The listing builds one solid part. Answer for the finished solid, in the listing's coordinates (mm). A direction names the side the tool comes from. Round coordinates to 2 decimals unless told otherwise and drop trailing zeros. Loops run counter-clockwise (first coordinate to the right, second up) from the corner with the lowest first, then second, coordinate; pieces in that order, holes last. Notation, with made-up numbers: (-35, 32.25) - (-14, 32.25) arc R29 ccw to (-14, 61.25) - close; hole circle Ø5 at (65, 47.25). An arc over 180 degrees is marked (long way). One line per item, written item: value.
```python
from build123d import *

# Parameters (mm, degrees)
F0_R     = 3
F0_R_2   = 1.5
F1_DEPTH = 25


with BuildPart() as f1:
    # F0 (on Front) → F1 (new body)
    with BuildSketch(Plane.XZ):
        with BuildLine():
            Line((14.5, 22.5), (-16.5, 22.5))
            ThreePointArc((-16.5, 22.5), (-17.9142135624, 21.9142135624), (-18.5, 20.5))
            Line((-18.5, 20.5), (-18.5, 17.6726558901))
            Line((-18.5, 17.6726558901), (-18.5, -20.5))
            ThreePointArc((-18.5, -20.5), (-17.9142135624, -21.9142135624), (-16.5, -22.5))
            Line((-16.5, -22.5), (-2.7271780287, -22.5))
            ThreePointArc((-2.7271780287, -22.5), (-3, -21.25), (-2.7271780287, -20))
            Line((-2.7271780287, -20), (-14, -20))
            ThreePointArc((-14, -20), (-14.7071067812, -19.7071067812), (-15, -19))
            Line((-15, -19), (-15, -15.5))
            Line((-15, -15.5), (-15, 2.5))
            ThreePointArc((-15, 2.5), (-14.4142135624, 3.9142135624), (-13, 4.5))
            Line((-13, 4.5), (-12, 4.5))
            ThreePointArc((-12, 4.5), (-10.5857864376, 5.0857864376), (-10, 6.5))
            Line((-10, 6.5), (-10, 8.1054256072))
            ThreePointArc((-10, 8.1054256072), (-9.6405519552, 9.2493614806), (-8.6914107177, 9.9821118409))
            Line((-8.6914107177, 9.9821118409), (6.3085892823, 15.5084276303))
            ThreePointArc((6.3085892823, 15.5084276303), (8.1439358734, 15.2722933519), (9, 13.6317413967))
            Line((9, 13.6317413967), (9, 2.5))
            ThreePointArc((9, 2.5), (9.2928932188, 1.7928932188), (10, 1.5))
            Line((10, 1.5), (13, 1.5))
            ThreePointArc((13, 1.5), (14.4142135624, 0.9142135624), (15, -0.5))
            Line((15, -0.5), (15, -15.5))
            ThreePointArc((15, -15.5), (14.9989931779, -15.5634529316), (14.9959737255, -15.6268419774))
            Line((14.9959737255, -15.6268419774), (14.8878943659, -19.0317264658))
            ThreePointArc((14.8878943659, -19.0317264658), (14.5841971496, -19.7182361958), (13.8883977769, -20))
            Line((13.8883977769, -20), (2.7271780287, -20))
            ThreePointArc((2.7271780287, -20), (2.9310010309, -20.6102868166), (3, -21.25))
            ThreePointArc((3, -21.25), (2.9310010309, -21.8897131834), (2.7271780287, -22.5))
            Line((2.7271780287, -22.5), (16.5, -22.5))
            ThreePointArc((16.5, -22.5), (17.9142135624, -21.9142135624), (18.5, -20.5))
            Line((18.5, -20.5), (18.5, 3.5))
            ThreePointArc((18.5, 3.5), (18.2071067812, 4.2071067812), (17.5, 4.5))
            ThreePointArc((17.5, 4.5), (16.7928932188, 4.7928932188), (16.5, 5.5))
            Line((16.5, 5.5), (16.5, 17.6726558901))
            Line((16.5, 17.6726558901), (16.5, 20.5))
            ThreePointArc((16.5, 20.5), (15.9142135624, 21.9142135624), (14.5, 22.5))
        make_face()
        with BuildLine():
            ThreePointArc((-12.5, 17.6726558901), (-15.5, 14.6726558901), (-18.5, 17.6726558901))
            ThreePointArc((-18.5, 17.6726558901), (-15.5, 20.6726558901), (-12.5, 17.6726558901))
        make_face(mode=Mode.SUBTRACT)
        with Locations((13.5, 17.6726558901)):
            Circle(F0_R, mode=Mode.SUBTRACT)
        with BuildLine():
            ThreePointArc((-2.7271780287, -20), (-3, -21.25), (-2.7271780287, -22.5))
            Line((-2.7271780287, -22.5), (-0.8291561976, -22.5))
            ThreePointArc((-0.8291561976, -22.5), (-1.5, -21.25), (-0.8291561976, -20))
            Line((-0.8291561976, -20), (-2.7271780287, -20))
        make_face()
        with BuildLine():
            Line((-0.8291561976, -22.5), (-2.7271780287, -22.5))
            ThreePointArc((-2.7271780287, -22.5), (0, -24.25), (2.7271780287, -22.5))
            Line((2.7271780287, -22.5), (0.8291561976, -22.5))
            ThreePointArc((0.8291561976, -22.5), (0, -22.75), (-0.8291561976, -22.5))
        make_face()
        with BuildLine():
            Line((0.8291561976, -22.5), (2.7271780287, -22.5))
            ThreePointArc((2.7271780287, -22.5), (2.9310010309, -21.8897131834), (3, -21.25))
            ThreePointArc((3, -21.25), (2.9310010309, -20.6102868166), (2.7271780287, -20))
            Line((2.7271780287, -20), (0.8291561976, -20))
            ThreePointArc((0.8291561976, -20), (1.3216910184, -20.5406814173), (1.5, -21.25))
            ThreePointArc((1.5, -21.25), (1.3216910184, -21.9593185827), (0.8291561976, -22.5))
        make_face()
        with BuildLine():
            ThreePointArc((2.7271780287, -20), (0, -18.25), (-2.7271780287, -20))
            Line((-2.7271780287, -20), (-0.8291561976, -20))
            ThreePointArc((-0.8291561976, -20), (0, -19.75), (0.8291561976, -20))
            Line((0.8291561976, -20), (2.7271780287, -20))
        make_face()
        with BuildLine():
            ThreePointArc((-12.5, 17.6726558901), (-15.5, 20.6726558901), (-18.5, 17.6726558901))
            ThreePointArc((-18.5, 17.6726558901), (-15.5, 14.6726558901), (-12.5, 17.6726558901))
        make_face()
        with Locations((-15.5, 17.6726558901)):
            Circle(F0_R_2, mode=Mode.SUBTRACT)
        with Locations((13.5, 17.6726558901)):
            Circle(F0_R)
        with Locations((13.5, 17.6726558901)):
            Circle(F0_R_2, mode=Mode.SUBTRACT)
    extrude(amount=F1_DEPTH)


solid = f1.part
```
1) A cutting plane is placed at A-A on x = 11. Give the vertices of the cut face in (y, z), and give its area (4 significant figures).
Final values:
outline: (-25, -22.5) - (0, -22.5) - (0, -20) - (-25, -20) - close; (-25, 1.5) - (0, 1.5) - (0, 22.5) - (-25, 22.5) - close
area: 587.5 mm2
2) Consider L1, parallel to Z at x = 11.5, y = -15.5; L2, parallel to X at y = -12, z = -5.5; L3, parallel to Z at x = 13.5, y = -14.75. Determine where each line is inside the solid, lowest interval first.
Final values:
L1: -22.5 to -20, 1.5 to 22.5
L2: -18.5 to -15, 15 to 18.5
L3: -22.5 to -20, 1.44 to 16.17, 19.17 to 22.5
3) For a pull along X with two mould halves and no side action, classify faces 5 (the flat face through (18.5, -12, -9)), 6 (the flat face through (11, -12, 1.5)), 7 (the flat face through (-10, -12, -22.5)) as released by +X, released by -X, zero draft, split by the parting line, or undercut.
Final values:
face 5: released by +X
face 6: undercut
face 7: zero draft
4) A cutting plane is placed at C-C on z = -4. Give the vertices of the cut face in (x, y), and give its area (3 significant figures).
Final values:
outline: (-18.5, -25) - (-15, -25) - (-15, 0) - (-18.5, 0) - close; (15, -25) - (18.5, -25) - (18.5, 0) - (15, 0) - close
area: 175 mm2
5) Each of these flat-tipped pins is pushed along its axis until it touches: pin 1 Ø15 at (x, y) = (-8.5, -17.5) entering from -Z; pin 2 Ø4.5 at (y, z) = (-8, 13) entering from +X; pin 3 Ø1.5 at (x, y) = (11.5, -10) entering from -Z. Where does it stop, or does it pass through?
Final values:
pin 1: z = -24.08
pin 2: x = 16.5
pin 3: z = -22.5
6) A cutting plane is placed at D-D on y = -21. Give the number of separate pieces and of enclosed holes in the cut face, and give its area (3 significant figures).
Final values:
separate pieces: 1
enclosed holes: 4
area: 743 mm2
7) A cutting plane is placed at B-B on z = 18.5. Give the vertices of the cut face in (x, y), and give its area (3 significant figures).
Final values:
outline: (-18.5, -25) - (-16.75, -25) - (-16.75, 0) - (-18.5, 0) - close; (-14.25, -25) - (12.25, -25) - (12.25, 0) - (-14.25, 0) - close; (14.75, -25) - (16.5, -25) - (16.5, 0) - (14.75, 0) - close
area: 750 mm2
8) For faces 1 (the flat face through (-18.5, -12, 0)), 2 (the flat face through (8, -12, -20)), 3 (the flat face through (10, -12, -22.5)), 4 (the flat face through (16.5, -12, 13)), determine the directions among +Z, -Z, +X, -X, +Y, -Y from which every point of the face is accessible in a straight line to the end or side of a thin tool.
Final values:
face 1: +Z, -Z, -X, +Y, -Y
face 2: +Y, -Y
face 3: -Z, +X, +Y, -Y
face 4: +Z, +X, +Y, -Y
